Autodesk Inventor part; units mm, degrees
ref_plane "YZ Plane" through (0, 0, 0) normal (1, 0, 0) x (0, 1, 0)
ref_plane "XZ Plane" through (0, 0, 0) normal (0, 1, 0) x (-1, 0, 0)
ref_plane "XY Plane" through (0, 0, 0) normal (0, 0, 1) x (1, 0, 0)
sketch "Sketch1" plane through (0, 0, 0) normal (0, 0, 1) x (1, 0, 0)
  circle A0 centre (0, 0) radius 19.05
  circle A1 centre (0, 0) radius 11.1125
  line L0 (0, 0) -> (0, -12.7)
  circle A2 centre (0, -12.7) radius 4.7625
  circle A3 centre (10.9985, 6.35) radius 4.7625
  circle A4 centre (-10.9985, 6.35) radius 4.7625
  dimension "d0" = 38.1
  dimension "d1" = 22.225
  dimension "d2" = 12.7
  dimension "d3" = 9.525
  dimension "d6" = 360
extrude "Extrusion1" add sketch "Sketch1" along normal blind 3.175 contours A0 | A3 A1 | A1 A3 | A2 A1 | A1 L0 A2 | A1 A2 L0 | A4 A1 | A1 A4
sketch "Sketch2" plane through (0, 0, 0) normal (1, 0, 0) x (0, 1, 0)
  line L0 (0, 0) -> (0, 19.3707)
  line L1 (19.05, 3.175) -> (-19.05, 3.175)
  line L2 (0, 3.175) -> (15.24, 3.175)
  line L3 (0, 3.175) -> (0, 6.35)
  line L4 (0, 6.35) -> (4.7625, 6.35)
  arc A0 (15.24, 3.175) -> (4.7625, 6.35) centre (1.074, -24.6976) ccw
  line L5 (4.7625, 6.35) -> (4.7625, 3.175)
  dimension "d10" = 15.24
  dimension "d11" = 3.175
  dimension "d12" = 4.7625
revolve "Revolution1" add sketch "Sketch2" angle 360 about axis through (0, 0, 3.175) along (0, 0, 1) contours L5 A0 L1
sketch "Sketch3" plane through (0, 0, 3.175) normal (0, 0, 1) x (1, 0, 0)
  line L0 (0, 0) -> (0, 9.525)
  circle A0 centre (0, 9.525) radius 3.175
  circle A1 centre (0, 9.525) radius 4.1275
  dimension "d14" = 9.525
  dimension "d15" = 6.35
  dimension "d16" = 8.255
extrude "Extrusion2" add sketch "Sketch3" along normal blind 3.175
sketch "Sketch4" plane through (0, 9.525, 6.35) normal (0, 0, 1) x (1, 0, 0)
  circle A0 centre (0, 0) radius 4.1275
  point P0 (0, -9.525)
extrude "Extrusion3" add sketch "Sketch4" along normal blind 1.27
extrude "Extrusion4" cut sketch "Sketch3" against normal through all contours A0
properties part number "SpurGear" material "ABS Plastic"
Source: CAD feature listing. Evaluate the final solid. Frame: model axes, mm. A direction names the side the tool comes from. Give positions to 0.01 mm unless a question says otherwise; leave off trailing zeros. Write each loop counter-clockwise with the first axis right and the second up, starting at its lowest first coordinate (ties: lowest second). Pieces come first, ordered by that corner, then holes. Notation, with made-up numbers: M -35.75,26 L 1.25,26 A20 cw 1.25,57 Z; hole C -21,-12.75 d10. An arc over 180 degrees is marked long. Answer as a JSON object with one key per item and string values.
Q1. Cut plane C-C, the plane x = 17.5. Return the cut outline in (y, z) (3 decimals).
Geometry check:
{"outline": "M -7.527,0 L 7.527,0 L 7.527,3.175 L -7.527,3.175 Z"}
Q2. Contact query for flat-ended pins moving along their axis: P1, Ø2, axis at y = -8, z = 3, coming from the +X side; P2, Ø2, axis at x = -8.5, z = 2.5, coming from the +Y side; P3, Ø1, axis at x = 0, y = 8, coming from the -Z side (3 decimals). Output: stop coordinate, or through.
Geometry check:
{"P1": "stops at x = 17.72", "P2": "stops at y = 17.51", "P3": "stops at z = 3.175"}
Q3. Access query for faces 1 (the face through (-5.036, 9.906, 1.565)), 2 (the face through (-0.688, 12.624, 5.549)), 3 (the face through (-0.895, 13.554, 6.158)). Directions: +Z, -Z, +X, -X, +Y, -Y. A direction counts if a zero-diameter tool reaches every point of the face in a straight line with its end or side. Return the directions, or none.
Geometry check:
{"face 1": "-Z", "face 2": "none", "face 3": "+Z"}
Q4. Mould query, pull axis X, two halves, no side actions, for faces 4 (the face through (-15.12, 11.59, 1.57)), 5 (the face through (-9.6, -5.6, 1.6)), 6 (the face through (-9, 13, 3.175)). Classes: +X half, -X half, draft (parallel to the pull), parting line (faces both ways), or undercut.
Geometry check:
{"face 4": "parting line", "face 5": "undercut", "face 6": "draft"}
Q5. Cut plane B-B, the plane x = 0.5. Count the separate pieces of the cut face and the enclosed holes in it, then the cut area to 3 significant figures.
Geometry check:
{"separate pieces": "2", "enclosed holes": "1", "area": "109 mm^2"}
Q6. Ray query, line 1 along X through (y, z) = (-8.5, 2); line 2 along X through (y, z) = (5, 2.75); line 3 along X through (y, z) = (6, 0.5). Return the intervals inside material, ascending.
Geometry check:
{"line 1": "x = -17.05 to -7.16, -2.25 to 2.25, 7.16 to 17.05", "line 2": "x = -18.38 to -6.43, 6.43 to 18.38", "line 3": "x = -18.08 to -6.25, 6.25 to 18.08"}
